Input: part model. Units: mm. Frame: model coordinates. A direction names the side the tool comes from. Give positions to 0.01 mm unless a question says otherwise; leave off trailing zeros. Write each loop counter-clockwise with the first axis right and the second up, starting at its lowest first coordinate (ties: lowest second). Pieces come first, ordered by that corner, then holes.
```python
from build123d import *

# Parameters (mm, degrees)
F3_R  = 6.35
F6_R  = 6.35
F9_R  = 6.35
F12_R = 6.35
F15_R = 6.35
F18_R = 6.35


with BuildPart() as f4:
    # F4: sweep along a path in F0
    with BuildLine(Plane.XY) as f4_path:
        Line((0, -165.1), (0, 165.1))
    # F3 (on plane+point) → F4 (sweep)
    with BuildSketch(Plane.XZ.offset(-165.1)):
        Circle(F3_R)
    sweep(path=f4_path.line)

    # F7: sweep along a path in F0
    with BuildLine(Plane.XY) as f7_path:
        Line((-165.1, 0), (165.1, 0))
    # F6 (on plane+point) → F7 (sweep)
    with BuildSketch(Plane.YZ.offset(165.1)):
        Circle(F6_R)
    sweep(path=f7_path.line)

    # F10: sweep along a path in F0
    with BuildLine(Plane.XY) as f10_path:
        Line((30.48, -142.8340719156), (30.48, 142.8340719156))
    # F9 (on plane+point) → F10 (sweep)
    with BuildSketch(Plane.XZ.offset(142.8340719156)):
        with Locations((30.48, 0)):
            Circle(F9_R)
    sweep(path=f10_path.line)

    # F13: sweep along a path in F0
    with BuildLine(Plane.XY) as f13_path:
        Line((60.96, -132.719557338), (60.96, 132.719557338))
    # F12 (on plane+point) → F13 (sweep)
    with BuildSketch(Plane.XZ.offset(132.719557338)):
        with Locations((60.96, 0)):
            Circle(F12_R)
    sweep(path=f13_path.line)

    # F16: sweep along a path in F0
    with BuildLine(Plane.XY) as f16_path:
        Line((91.44, -113.8829614121), (91.44, 113.8829614121))
    # F15 (on plane+point) → F16 (sweep)
    with BuildSketch(Plane.XZ.offset(113.8829614121)):
        with Locations((91.44, 0)):
            Circle(F15_R)
    sweep(path=f16_path.line)

    # F19: sweep along a path in F0
    with BuildLine(Plane.XY) as f19_path:
        Line((121.92, -80.4121638808), (121.92, 80.4121638808))
    # F18 (on plane+point) → F19 (sweep)
    with BuildSketch(Plane.XZ.offset(80.4121638808)):
        with Locations((121.92, 0)):
            Circle(F18_R)
    sweep(path=f19_path.line)

    # F20: F4 across plane


with BuildPart() as f4_1:
    add(f4.part)
    add(f4.part.mirror(Plane.YZ))


solid = f4_1.part
```
Q1. Access query for faces 1 (the cylindrical face through (-45.93, -4.68, 4.29)), 2 (the flat face through (-31, -142.834, 0)), 3 (the cylindrical face through (67.017, 67.289, -1.907)), 4 (the flat face through (-31, 142.834, 0)). Directions: +Z, -Z, +X, -X, +Y, -Y. A direction counts if a zero-diameter tool reaches every point of the face in a straight line with its end or side. Return the directions, or none.
Q2. Section C-C, the plane x = 43. Return the cut outline in (y, z), then the cut area to 3 significant figures.
Q3. Mould query, pull axis X, two halves, no side actions, for faces 5 (the flat face through (-61, 132.72, 0)), 6 (the cylindrical face through (-127.977, -39.643, -1.907)). Classes: +X half, -X half, draft (parallel to the pull), parting line (faces both ways), or undercut.
Q4. Material intervals for line 1 along X through (y, z) = (-114.5, -2.5); line 2 along Y through (x, z) = (102, -0.75); line 3 along Y through (x, z) = (-26, 2), sorted ascending.
Q5. Section B-B, the plane y = -90.5. Return the cut outline in (x, z), then the cut area to 3 significant figures.
Q6. Pin query (flat end, axial travel): pin 1 (4 mm diameter, centred on y = -87, z = -0.5, fed in from -X); pin 2 (6.5 mm diameter, centred on x = 63.5, z = 2.5, fed in from +Y); pin 3 (6.5 mm diameter, centred on x = -31, z = 0.5, fed in from +Y). Return the tip coordinate at first contact, or that it passes through.
Q7. Section A-A, the plane y = 22. Give the number of separate pieces and of enclosed holes in the cut face, then the cut area to 3 significant figures.
Solutions:
1. face 1: none
1. face 2: +Z, -Z, -X, -Y
1. face 3: +Y
1. face 4: +Z, -Z, -X, +Y
2. outline: circle Ø12.7 at (0, 0)
2. area: 127 mm2
3. face 5: draft
3. face 6: undercut
4. line 1: x = -66.8 to -55.12, -36.32 to -24.64, -5.84 to 5.84, 24.64 to 36.32, 55.12 to 66.8
4. line 2: y = -6.31 to 6.31
4. line 3: y = -142.83 to 142.83
5. outline: circle Ø12.7 at (-91.44, 0); circle Ø12.7 at (-60.96, 0); circle Ø12.7 at (-30.48, 0); circle Ø12.7 at (0, 0); circle Ø12.7 at (30.48, 0); circle Ø12.7 at (60.96, 0); circle Ø12.7 at (91.44, 0)
5. area: 887 mm2
6. pin 1: stops at x = -97.79
6. pin 2: stops at y = 132.72
6. pin 3: stops at y = 142.83
7. separate pieces: 9
7. enclosed holes: 0
7. area: 1,140 mm2
